Geometry check sheet. Reference: drawing and pictorial views, mm from the part's lowest x, y, z. Coordinates: 2 decimals unless noted, no trailing zeros. Loops run counter-clockwise (first coordinate to the right, second up) from the corner with the lowest first, then second, coordinate; pieces in that order, holes last. Notation, with made-up numbers: (-21, 80.25) - (20, 80.25) arc R8 ccw to (20, 85.25) - close; hole circle Ø4 at (47, 78). An arc over 180 degrees is marked (long way). Use a Markdown table: item, result. Add a question column.
1) Thickness scan on line 1 (X direction, y = 23.5, z = 1.25); line 2 (X direction, y = 3, z = 1.5); line 3 (Y direction, x = 340.5, z = 0.3) (3 decimals). Record the ranges inside material, lowest first.
2) Go/stop test with flat-tipped pins: P1, Ø1.6, axis at y = 55.5, z = 2, coming from the -X side; P2, Ø1.6, axis at y = 56.5, z = 1, coming from the +X side; P3, Ø1, axis at x = 151.5, z = 1.5, coming from the -Y side (3 decimals). Record where each tip stops, or that it passes through.
3) Sectioned sample at A-A, the plane y = 16.5. Enter the section's corners in (x, z) (3 decimals), then the cut area to 3 significant figures.
4) Sectioned sample at B-B, the plane x = 74.5. Enter the section's corners in (y, z) (3 decimals).
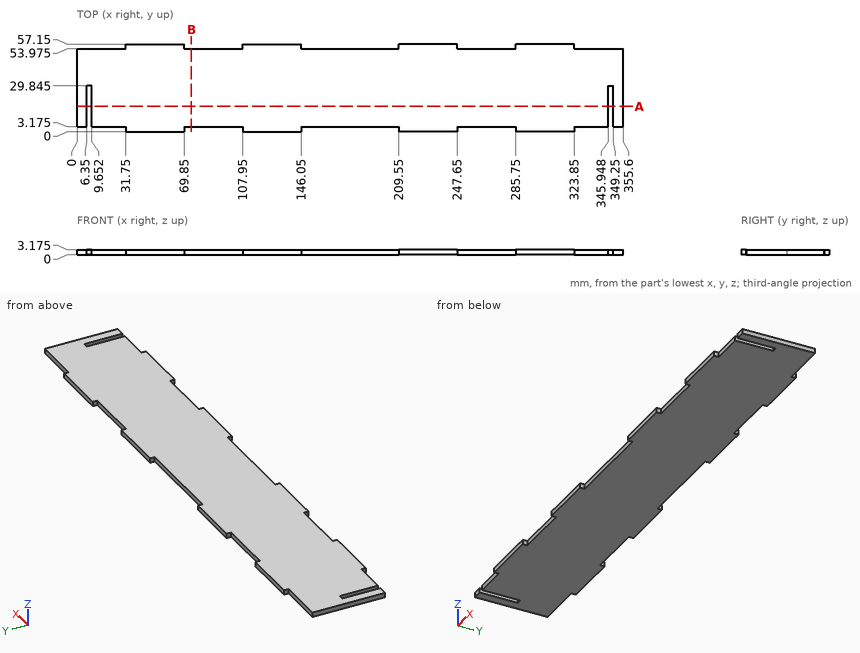
Solved:
| question | item | result |
|---|---|---|
| 1 | line 1 | x = 0 to 6.35, 9.65 to 345.95, 349.25 to 355.6 |
| 1 | line 2 | x = 31.75 to 69.85, 107.95 to 146.05, 209.55 to 247.65, 285.75 to 323.85 |
| 1 | line 3 | y = 3.175 to 53.975 |
| 2 | P1 | stops at x = 31.75 |
| 2 | P2 | stops at x = 323.85 |
| 2 | P3 | stops at y = 3.175 |
| 3 | outline | (0, 0) - (6.35, 0) - (6.35, 3.175) - (0, 3.175) - close; (9.652, 0) - (345.948, 0) - (345.948, 3.175) - (9.652, 3.175) - close; (349.25, 0) - (355.6, 0) - (355.6, 3.175) - (349.25, 3.175) - close |
| 3 | area | 1,110 mm2 |
| 4 | outline | (3.175, 0) - (53.975, 0) - (53.975, 3.175) - (3.175, 3.175) - close |
